The listing builds one solid part. Answer for the finished solid, in the listing's coordinates (mm). Face numbers are marked on the shaded views. Give positions to 0.01 mm unless a question says otherwise; leave off trailing zeros. Write each loop counter-clockwise with the first axis right and the second up, starting at its lowest first coordinate (ties: lowest second). Pieces come first, ordered by that corner, then holes. Notation, with made-up numbers: M -35.5,-10 L -27.5,-10 A12 cw -27.5,-3 Z; hole C -15.5,10.5 d1. An arc over 180 degrees is marked long. Return JSON: item names as keys, results as strings.
Autodesk Inventor part; units mm, degrees
ref_plane "YZ Plane" through (0, 0, 0) normal (1, 0, 0) x (0, 1, 0)
ref_plane "XZ Plane" through (0, 0, 0) normal (0, 1, 0) x (-1, 0, 0)
ref_plane "XY Plane" through (0, 0, 0) normal (0, 0, 1) x (1, 0, 0)
sketch "スケッチ1" plane through (0, 0, 0) normal (0, 0, 1) x (1, 0, 0)
  arc A0 (0, 10) -> (7.1414, -7) centre (0, 0) ccw
  circle A1 centre (0, 0) radius 7 construction
  circle A2 centre (0, 7) radius 1.1
  circle A3 centre (0, 0) radius 7 construction
  circle A4 centre (-4.9497, 4.9497) radius 1.1
  circle A5 centre (0, 0) radius 7 construction
  circle A6 centre (-7, 0) radius 1.1
  circle A7 centre (0, 0) radius 7 construction
  circle A8 centre (-4.9497, -4.9497) radius 1.1
  circle A9 centre (0, 0) radius 7 construction
  circle A10 centre (0, -7) radius 1.1
  circle A11 centre (0, 0) radius 7 construction
  circle A12 centre (4.9497, -4.9497) radius 1.1
  circle A13 centre (0, 0) radius 7 construction
  circle A14 centre (7, 0) radius 1.1
  circle A15 centre (0, 0) radius 7 construction
  circle A16 centre (4.9497, 4.9497) radius 1.1
  line L0 (0, 10) -> (28, 25)
  circle A17 centre (0, 0) radius 5.1
  line L1 (43, -7) -> (43, 25)
  line L2 (7.1414, -7) -> (43, -7)
  line L3 (43, -7) -> (28, -7)
  line L4 (28, -7) -> (28, 25) construction
  line L5 (28, 25) -> (43, 25)
  line L6 (35.5, 25) -> (35.5, -7) construction
  line L7 (43, 9) -> (28, 9) construction
  circle A18 centre (35.5, 22) radius 1.6
  circle A19 centre (35.5, -4) radius 1.6
  line L8 (0, 0) -> (-10, 0) construction
  circle A20 centre (35.5, 22) radius 3 construction
  circle A21 centre (35.5, -4) radius 3 construction
  circle A22 centre (35.5, 15) radius 1.6 construction
  circle A23 centre (35.5, 15) radius 3 construction
  circle A24 centre (35.5, 3) radius 1.6 construction
  circle A25 centre (35.5, 3) radius 3 construction
  line L9 (0, 0) -> (0, 10) construction
  dimension "d1" = 14
  dimension "d0" = 20
  dimension "d2" = 2.2
  dimension "d5" = 360
  dimension "d7" = 10.2
  dimension "d11" = 15
  dimension "d12" = 90
  dimension "d13" = 3.2
  dimension "d14" = 3.2
  dimension "d15" = 35.8586
  dimension "d16" = 7
  dimension "d18" = 6
  dimension "d19" = 6
  dimension "d20" = 3.2
  dimension "d21" = 6
  dimension "d22" = 6
  dimension "d23" = 32
extrude "押し出し1" add sketch "スケッチ1" along normal blind 1.5
properties part number "サーボ支え板A_アルミ(A2017)_t1.5" material "アルミニウム 6061"
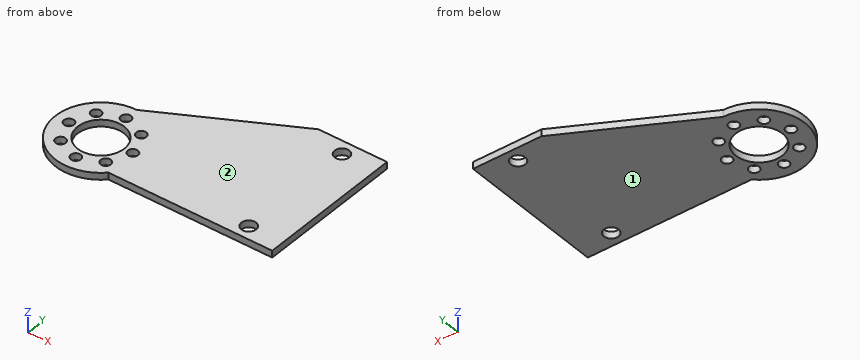
Item 1: A cutting plane is placed at B-B, the plane y = 0. Write down the section's boundary in (x, z), plus the area to 3 significant figures.
Geometry results:
{"outline": "M -10,0 L -8.1,0 L -8.1,1.5 L -10,1.5 Z; M -5.9,0 L -5.1,0 L -5.1,1.5 L -5.9,1.5 Z; M 5.1,0 L 5.9,0 L 5.9,1.5 L 5.1,1.5 Z; M 8.1,0 L 43,0 L 43,1.5 L 8.1,1.5 Z", "area": "57.6 mm2"}
Item 2: A cutting plane is placed at D-D, the plane z = 0.3. Count the separate pieces of the cut face and the enclosed holes in it, plus the area to 3 significant figures.
Geometry results:
{"separate pieces": "1", "enclosed holes": "11", "area": "1,210 mm2"}
Item 3: A cutting plane is placed at C-C, the plane x = -2. Write down the section's boundary in (y, z).
Geometry results:
{"outline": "M -9.8,0 L -4.69,0 L -4.69,1.5 L -9.8,1.5 Z; M 4.69,0 L 9.8,0 L 9.8,1.5 L 4.69,1.5 Z"}
Item 4: Given pin 1 Ø1.8 at (x, y) = (0, 7) entering from -Z, flat-ended and moving along its own axis, determine where the tip first touches the part or whether it passes through.
Geometry results:
{"pin 1": "passes through"}
Item 5: A cutting plane is placed at A-A, the plane y = 22. Write down the section's boundary in (x, z).
Geometry results:
{"outline": "M 22.4,0 L 33.9,0 L 33.9,1.5 L 22.4,1.5 Z; M 37.1,0 L 43,0 L 43,1.5 L 37.1,1.5 Z"}
Item 6: Find the intervals of material crossed by line 1 (Y direction, x = 0, z = 0.7); line 2 (Y direction, x = 35.5, z = 1.15); line 3 (Y direction, x = 7, z = 0.9), in increasing order.
Geometry results:
{"line 1": "y = -10 to -8.1, -5.9 to -5.1, 5.1 to 5.9, 8.1 to 10", "line 2": "y = -7 to -5.6, -2.4 to 20.4, 23.6 to 25", "line 3": "y = -7.14 to -1.1, 1.1 to 13.75"}
Item 7: Determine the mould class of the marked faces 1 and 2 for opening direction Z: +Z half, -Z half, draft (parallel to the pull), parting line (faces both ways), or undercut.
Geometry results:
{"face 1": "-Z half", "face 2": "+Z half"}
